For this review, take the finished solid that the model builds, in its own axes (mm). A direction names the side the tool comes from. Round coordinates to 2 decimals unless told otherwise and drop trailing zeros. Order: outer loops, then holes, each group sorted by start corner. A loop starts at its lowest first (then second) coordinate and runs counter-clockwise, first axis right, second up. Notation, with made-up numbers: M 54.5,37 L 88.5,37 A36 cw 88.5,71 Z; hole C 20.25,33.25 d3. An arc over 180 degrees is marked long. Answer as a JSON object with one key per item and string values.
Autodesk Inventor part; units mm, degrees
ref_plane "YZ Plane" through (0, 0, 0) normal (1, 0, 0) x (0, 1, 0)
ref_plane "XZ Plane" through (0, 0, 0) normal (0, 1, 0) x (-1, 0, 0)
ref_plane "XY Plane" through (0, 0, 0) normal (0, 0, 1) x (1, 0, 0)
sketch "草圖1" plane through (0, 0, 0) normal (0, 1, 0) x (-1, 0, 0)
  circle A0 centre (0, 0) radius 40
  dimension "d0" = 80
extrude "擠出1" add sketch "草圖1" along normal blind 10
sketch "草圖2" plane through (0, 10, 0) normal (0, 1, 0) x (1, 0, 0)
  circle A0 centre (0, 0) radius 12.5
  dimension "d3" = 25
extrude "擠出2" add sketch "草圖2" along normal blind 20
sketch "草圖3" plane through (0, 30, 0) normal (0, 1, 0) x (1, 0, 0)
  circle A0 centre (0, 0) radius 6
  dimension "d6" = 12
extrude "擠出3" cut sketch "草圖3" against normal blind 60
sketch "草圖4" plane through (0, 10, 0) normal (0, 1, 0) x (1, 0, 0)
  circle A0 centre (0, 0) radius 6
  circle A1 centre (0, 0) radius 26 construction
  circle A2 centre (26, 0) radius 5
  line L0 (0, 0) -> (48.0653, 0)
  dimension "d9" = 52
  dimension "d10" = 10
extrude "擠出4" cut sketch "草圖4" against normal blind 60 contours A2 L0 | L0 A2
pattern_circular "環形陣列1" count 6 over 360 about axis through (0, 30, 0) along (0, -1, 0) of "擠出4"
properties part number "練習三"
1) Mouldability with a two-part tool opening along Z and no side actions: class faces 3 (the cylindrical face through (-10.31, 5.07, -26.73)), 4 (the cylindrical face through (8.67, 4.93, 39.05)), 5 (the flat face through (-3, 30, 5.4)) as +Z half, -Z half, draft (parallel to the pull), parting line (faces both ways), or undercut.
Geometry check:
{"face 3": "undercut", "face 4": "parting line", "face 5": "draft"}
2) Add section A-A on z = 0. State the section outline as (x, y) points.
Geometry check:
{"outline": "M -40,0 L -31,0 L -31,10 L -40,10 Z; M -21,0 L -6,0 L -6,30 L -12.5,30 L -12.5,10 L -21,10 Z; M 6,0 L 21,0 L 21,10 L 12.5,10 L 12.5,30 L 6,30 Z; M 31,0 L 40,0 L 40,10 L 31,10 Z"}
3) Add section B-B on x = 0. State the section outline as (y, z) points.
Geometry check:
{"outline": "M 0,-40 L 10,-40 L 10,-12.5 L 30,-12.5 L 30,-6 L 0,-6 Z; M 0,6 L 30,6 L 30,12.5 L 10,12.5 L 10,40 L 0,40 Z"}
4) Insertion check: P1, Ø10, axis at y = 18, z = 13, coming from the +X side; P2, Ø2, axis at x = 29, z = 1, coming from the -Y side; P3, Ø4, axis at x = 31, y = 8, coming from the -Z side; P4, Ø6, axis at x = -3, y = 3.5, coming from the +Z side. Each pin has a flat end and moves straight along its axis. Give the tip position at first contact, or say it passes through.
Geometry check:
{"P1": "stops at x = 9.6", "P2": "passes through", "P3": "stops at z = -27.55", "P4": "stops at z = 40"}
5) For L1, parallel to Z at x = 0, y = 6.5; L2, parallel to X at y = 6, z = -1; L3, parallel to Z at x = 13, y = 7.5, list the stretches that pass through material, from the lowest coordinate up.
Geometry check:
{"L1": "z = -40 to -6, 6 to 40", "L2": "x = -39.99 to -30.9, -21.1 to -5.92, 5.92 to 21.1, 30.9 to 39.99", "L3": "z = -37.83 to -27.52, -17.52 to 17.52, 27.52 to 37.83"}
6) Machinability: for faces 1 (the flat face through (9, 10, 9)), 2 (the flat face through (-8, 0, 1)), which of the approach directions +Z, -Z, +X, -X, +Y, -Y give a long, thin tool a straight path to every point of the face, cutting with its end or side? Answer none if there is none.
Geometry check:
{"face 1": "+Y", "face 2": "+Z, -Z, +X, -X, -Y"}
7) Add section D-D on x = -13.5. State the section outline as (y, z) points.
Geometry check:
{"outline": "M 0,-37.65 L 10,-37.65 L 10,-27.49 L 0,-27.49 Z; M 0,-17.54 L 10,-17.54 L 10,17.54 L 0,17.54 Z; M 0,27.49 L 10,27.49 L 10,37.65 L 0,37.65 Z"}
